Here's how the part is built. I have some questions about the finished solid (model axes, mm). Face numbers are marked on the shaded views. A direction names the side the tool comes from. Round coordinates to 2 decimals unless told otherwise and drop trailing zeros. Loops run counter-clockwise (first coordinate to the right, second up) from the corner with the lowest first, then second, coordinate; pieces in that order, holes last. Notation, with made-up numbers: M 29.5,0 L 64.5,0 A12 ccw 64.5,9 Z; hole C 56,21.25 d7. An arc over 180 degrees is marked long. Answer as CSV lines item,"result".
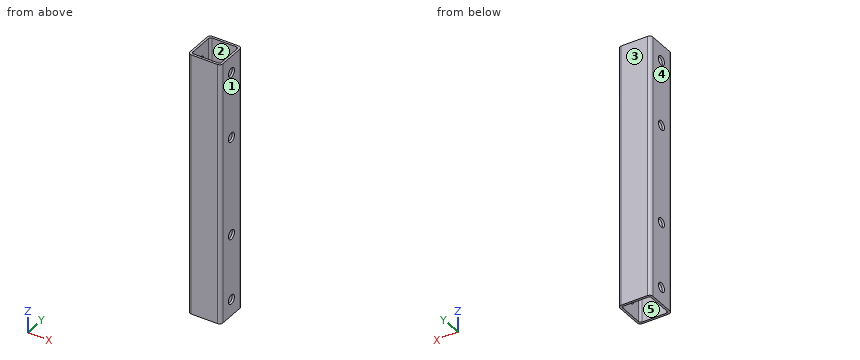
```python
from build123d import *

# Parameters (mm, degrees)
EXTRUDE_1_DEPTH     = 240
SKETCH_2_R          = 4.25
CUT_EXTRUDE_1_DEPTH = 244.721152139


with BuildPart() as part:
    # Эскиз1 → Бобышка-Вытянуть1 (new body)
    with BuildSketch(Plane.XY):
        with BuildLine():
            Line((-12, 30), (12, 30))
            ThreePointArc((12, 30), (14.121320344, 29.121320344), (15, 27))
            Line((15, 27), (15, 3))
            ThreePointArc((15, 3), (14.121320344, 0.878679656), (12, 0))
            Line((12, 0), (-12, 0))
            ThreePointArc((-12, 0), (-14.121320344, 0.878679656), (-15, 3))
            Line((-15, 3), (-15, 27))
            ThreePointArc((-15, 27), (-14.121320344, 29.121320344), (-12, 30))
        make_face()
        with BuildLine():
            Line((-11, 28), (11, 28))
            ThreePointArc((11, 28), (12.414213562, 27.414213562), (13, 26))
            Line((13, 26), (13, 4))
            ThreePointArc((13, 4), (12.414213562, 2.585786438), (11, 2))
            Line((11, 2), (-11, 2))
            ThreePointArc((-11, 2), (-12.414213562, 2.585786438), (-13, 4))
            Line((-13, 4), (-13, 26))
            ThreePointArc((-13, 26), (-12.414213562, 27.414213562), (-11, 28))
        make_face(mode=Mode.SUBTRACT)
    extrude(amount=EXTRUDE_1_DEPTH)

    # Эскиз2 → Вырез-Вытянуть1 (cut, through all)
    with BuildSketch(Plane(origin=(15, 0, 0), x_dir=(0, 0, -1), z_dir=(1, 0, 0))):
        with Locations(Location((-225, 15, 0), (0, 0, 90))):
            Circle(SKETCH_2_R)
        with Locations(Location((-165, 15, 0), (0, 0, 90))):
            Circle(SKETCH_2_R)
        with Locations(Location((-75, 15, 0), (0, 0, 90))):
            Circle(SKETCH_2_R)
        with Locations(Location((-15, 15, 0), (0, 0, 90))):
            Circle(SKETCH_2_R)
    extrude(amount=-CUT_EXTRUDE_1_DEPTH, mode=Mode.SUBTRACT)


solid = part.part
```
1. For P1, Ø7, axis at y = 15, z = 15, coming from the +X side; P2, Ø1.5, axis at x = 7.5, z = 179.5, coming from the -Y side, each with a flat end and sliding along its axis, tell me the tip position at first contact or that it passes through.
Evaluation:
P1,"passes through"
P2,"stops at y = 0"
2. We'd pull the mould along X, two halves only. Please class the marked faces 3, 4 and 5: pulls with the +X half, pulls with the -X half, needs draft (parallel to the pull), parting line crosses it, or undercut.
Evaluation:
face 3,"needs draft"
face 4,"pulls with the -X half"
face 5,"undercut"
3. I want a section at A-A, the plane y = 21.5. Please give me the cut outline in (x, z).
Evaluation:
outline,"M -15,0 L -13,0 L -13,240 L -15,240 Z; M 13,0 L 15,0 L 15,240 L 13,240 Z"
4. I want a section at B-B, the plane z = 147.5. Please give me the cut outline in (x, y).
Evaluation:
outline,"M -15,3 A3 ccw -12,0 L 12,0 A3 ccw 15,3 L 15,27 A3 ccw 12,30 L -12,30 A3 ccw -15,27 Z; hole M -13,4 A2 ccw -11,2 L 11,2 A2 ccw 13,4 L 13,26 A2 ccw 11,28 L -11,28 A2 ccw -13,26 Z"
5. I want a section at C-C, the plane x = 7. Please give me the cut outline in (y, z).
Evaluation:
outline,"M 0,0 L 2,0 L 2,240 L 0,240 Z; M 28,0 L 30,0 L 30,240 L 28,240 Z"
6. Which directions (+Z, -Z, +X, -X, +Y, -Y) give clear straight access to the entire face, cutting with the end or side of a thin tool? Please do the marked faces 1 and 2.
Evaluation:
face 1,"+Z, -Z, +X, +Y, -Y"
face 2,"+Z, -Z"
7. If I drill on line 1 (Z direction, x = 14.45, y = 15); line 2 (X direction, y = 7.5, z = 99.5); line 3 (Y direction, x = 2.5, z = 197), over which ranges is the centre line in solid material (lowest first)? Write a range as [from, to].
Evaluation:
line 1,"z = [0, 10.75], [19.25, 70.75], [79.25, 160.75], [169.25, 220.75], [229.25, 240]"
line 2,"x = [-15, -13], [13, 15]"
line 3,"y = [0, 2], [28, 30]"
